Part model, mm, in its own coordinate system. Face numbers are marked on the shaded views. A direction names the side the tool comes from. Round coordinates to 2 decimals unless told otherwise and drop trailing zeros. Write each loop counter-clockwise with the first axis right and the second up, starting at its lowest first coordinate (ties: lowest second). Pieces come first, ordered by that corner, then holes. Notation, with made-up numbers: (-29, 59) -> (-13, 59) arc R19 ccw to (-13, 76) -> close; hole circle Ø5 at (67, 84). An arc over 180 degrees is marked (long way). Return JSON: item names as keys, results as strings. Group by question number.
```python
from build123d import *

# Parameters (mm, degrees)
F1_DEPTH = 25


with BuildPart() as f1:
    # F0 (on Top) → F1 (new body)
    with BuildSketch(Plane.XY):
        with BuildLine():
            ThreePointArc((30, -68.7386354243), (62.7495019901, -41.0791918129), (75, 0))
            ThreePointArc((75, 0), (-41.0791918129, 62.7495019901), (-30, -68.7386354243))
            Line((-30, -68.7386354243), (-14.3843060635, -20))
            Line((-14.3843060635, -20), (-33.1410161514, -20))
            ThreePointArc((-33.1410161514, -20), (-35.9400542571, -20.75), (-33.8910161514, -18.7009618943))
            Line((-33.8910161514, -18.7009618943), (-28.8675134595, -10))
            Line((-28.8675134595, -10), (-32.3247935798, -10))
            ThreePointArc((-32.3247935798, -10), (-34.8854537516, -11.0606601718), (-33.8247935798, -8.5))
            Line((-33.8247935798, -8.5), (-33.8247935798, 8.5))
            ThreePointArc((-33.8247935798, 8.5), (-34.8854537516, 11.0606601718), (-32.3247935798, 10))
            Line((-32.3247935798, 10), (-17.3205080757, 10))
            Line((-17.3205080757, 10), (-0.75, 38.7009618943))
            ThreePointArc((-0.75, 38.7009618943), (-0.75, 41.2990381057), (1.5, 40))
            ThreePointArc((1.5, 40), (1.2990381057, 39.25), (0.75, 38.7009618943))
            Line((0.75, 38.7009618943), (17.3205080757, 10))
            Line((17.3205080757, 10), (32.3247935798, 10))
            ThreePointArc((32.3247935798, 10), (33.8247935798, 11.5), (35.3247935798, 10))
            ThreePointArc((35.3247935798, 10), (34.8854537516, 8.9393398282), (33.8247935798, 8.5))
            Line((33.8247935798, 8.5), (33.8247935798, -8.5))
            ThreePointArc((33.8247935798, -8.5), (34.8854537516, -8.9393398282), (35.3247935798, -10))
            ThreePointArc((35.3247935798, -10), (33.8247935798, -11.5), (32.3247935798, -10))
            Line((32.3247935798, -10), (28.8675134595, -10))
            Line((28.8675134595, -10), (33.8910161514, -18.7009618943))
            ThreePointArc((33.8910161514, -18.7009618943), (35.3910161514, -18.7009618943), (36.1410161514, -20))
            ThreePointArc((36.1410161514, -20), (34.6410161514, -21.5), (33.1410161514, -20))
            Line((33.1410161514, -20), (14.3843060635, -20))
            Line((14.3843060635, -20), (30, -68.7386354243))
        make_face()
        with BuildLine():
            Line((11.1803398875, -10), (14.3843060635, -20))
            Line((14.3843060635, -20), (33.1410161514, -20))
            ThreePointArc((33.1410161514, -20), (33.3419780457, -19.25), (33.8910161514, -18.7009618943))
            Line((33.8910161514, -18.7009618943), (28.8675134595, -10))
            Line((28.8675134595, -10), (11.1803398875, -10))
        make_face()
        with BuildLine():
            Line((-33.1410161514, -20), (-14.3843060635, -20))
            Line((-14.3843060635, -20), (-11.1803398875, -10))
            Line((-11.1803398875, -10), (-28.8675134595, -10))
            Line((-28.8675134595, -10), (-33.8910161514, -18.7009618943))
            ThreePointArc((-33.8910161514, -18.7009618943), (-33.3419780457, -19.25), (-33.1410161514, -20))
        make_face()
        with BuildLine():
            Line((-32.3247935798, -10), (-28.8675134595, -10))
            Line((-28.8675134595, -10), (-17.3205080757, 10))
            Line((-17.3205080757, 10), (-32.3247935798, 10))
            ThreePointArc((-32.3247935798, 10), (-32.764133408, 8.9393398282), (-33.8247935798, 8.5))
            Line((-33.8247935798, 8.5), (-33.8247935798, -8.5))
            ThreePointArc((-33.8247935798, -8.5), (-32.764133408, -8.9393398282), (-32.3247935798, -10))
        make_face()
        with BuildLine():
            Line((-17.3205080757, 10), (-11.1803398875, 10))
            ThreePointArc((-11.1803398875, 10), (0, 15), (11.1803398875, 10))
            Line((11.1803398875, 10), (17.3205080757, 10))
            Line((17.3205080757, 10), (0.75, 38.7009618943))
            ThreePointArc((0.75, 38.7009618943), (0, 38.5), (-0.75, 38.7009618943))
            Line((-0.75, 38.7009618943), (-17.3205080757, 10))
        make_face()
        with BuildLine():
            Line((17.3205080757, 10), (28.8675134595, -10))
            Line((28.8675134595, -10), (32.3247935798, -10))
            ThreePointArc((32.3247935798, -10), (32.764133408, -8.9393398282), (33.8247935798, -8.5))
            Line((33.8247935798, -8.5), (33.8247935798, 8.5))
            ThreePointArc((33.8247935798, 8.5), (32.764133408, 8.9393398282), (32.3247935798, 10))
            Line((32.3247935798, 10), (17.3205080757, 10))
        make_face()
        with BuildLine():
            ThreePointArc((15, 0), (14.0125853844, -5.3523313466), (11.1803398875, -10))
            Line((11.1803398875, -10), (28.8675134595, -10))
            Line((28.8675134595, -10), (17.3205080757, 10))
            Line((17.3205080757, 10), (11.1803398875, 10))
            ThreePointArc((11.1803398875, 10), (14.0125853844, 5.3523313466), (15, 0))
        make_face()
        with BuildLine():
            ThreePointArc((-11.1803398875, 10), (-15, 0), (-11.1803398875, -10))
            Line((-11.1803398875, -10), (11.1803398875, -10))
            ThreePointArc((11.1803398875, -10), (14.0125853844, -5.3523313466), (15, 0))
            ThreePointArc((15, 0), (14.0125853844, 5.3523313466), (11.1803398875, 10))
            Line((11.1803398875, 10), (-11.1803398875, 10))
        make_face()
        with BuildLine():
            Line((-28.8675134595, -10), (-11.1803398875, -10))
            ThreePointArc((-11.1803398875, -10), (-15, 0), (-11.1803398875, 10))
            Line((-11.1803398875, 10), (-17.3205080757, 10))
            Line((-17.3205080757, 10), (-28.8675134595, -10))
        make_face()
        with BuildLine():
            ThreePointArc((11.1803398875, 10), (0, 15), (-11.1803398875, 10))
            Line((-11.1803398875, 10), (11.1803398875, 10))
        make_face()
        with BuildLine():
            Line((11.1803398875, -10), (-11.1803398875, -10))
            ThreePointArc((-11.1803398875, -10), (0, -15), (11.1803398875, -10))
        make_face()
        with BuildLine():
            Line((-11.1803398875, -10), (-14.3843060635, -20))
            Line((-14.3843060635, -20), (14.3843060635, -20))
            Line((14.3843060635, -20), (11.1803398875, -10))
            ThreePointArc((11.1803398875, -10), (0, -15), (-11.1803398875, -10))
        make_face()
    extrude(amount=F1_DEPTH)


solid = f1.part
```
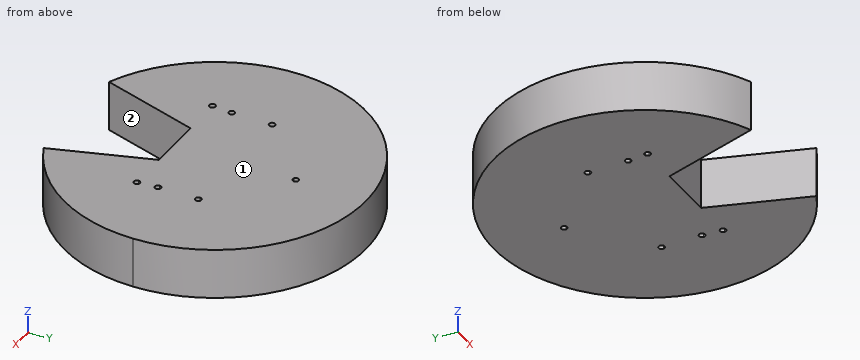
Item 1: Which spindle directions (+Z, -Z, +X, -X, +Y, -Y) get a long thin tool onto all of the face, cutting with end or side? Do the marked faces 1 and 2. Say none if no direction does.
Item 2: Cut at D-D (y = 14.5). Write the cut outline in (x, z).
Item 3: Cut at A-A (z = 7.5). Write the cut outline in (x, y), then the cut area to 3 significant figures.
Item 4: Flat gauge pins, fed straight in: P1, Ø1.5, axis at y = -50, z = 12, coming from the +X side; P2, Ø8, axis at x = 48, z = 18.5, coming from the +Y side; P3, Ø3, axis at y = 13.5, z = 8, coming from the +X side. Where does each tip first touch, or does it go through?
Item 5: Cut at C-C (x = -25). Write the cut outline in (y, z).
Item 6: Wall check: L1, parallel to Y at x = 0, z = 11; L2, parallel to X at y = -10, z = 19.75; L3, parallel to Y at x = 32.5, z = 7. Give the ranges that are in metal, low to high.
Item 7: Cut at B-B (y = -53.5). Write the cut outline in (x, z).
Checks:
{
 "1": {"face 1": "+Z, +X, -X, +Y, -Y", "face 2": "+Z, -Z, -Y"},
 "2": {"outline": "(-73.58, 0) -> (73.58, 0) -> (73.58, 25) -> (-73.58, 25) -> close"},
 "3": {"outline": "(-30, -68.74) -> (-14.38, -20) -> (14.38, -20) -> (30, -68.74) arc R75 ccw (long way) to start; hole circle Ø3 at (-34.64, -20); hole circle Ø3 at (-33.82, -10); hole circle Ø3 at (-33.82, 10); hole circle Ø3 at (0, 40); hole circle Ø3 at (33.82, -10); hole circle Ø3 at (33.82, 10); hole circle Ø3 at (34.64, -20)", "area": "15,200 mm2"},
 "4": {"P1": "stops at x = 56.56", "P2": "stops at y = 60.74", "P3": "stops at x = 74.03"},
 "5": {"outline": "(-53.13, 0) -> (70.71, 0) -> (70.71, 25) -> (-53.13, 25) -> close"},
 "6": {"L1": "y = -20 to 38.5, 41.5 to 75", "L2": "x = -74.33 to -35.32, -32.32 to 32.32, 35.32 to 74.33", "L3": "y = -67.59 to -10.7, -9.3 to 9.3, 10.7 to 67.59"},
 "7": {"outline": "(-52.56, 0) -> (-25.12, 0) -> (-25.12, 25) -> (-52.56, 25) -> close; (25.12, 0) -> (52.56, 0) -> (52.56, 25) -> (25.12, 25) -> close"}
}
